from build123d import *

# Parameters (mm, degrees)
SKETCH_1_W          = 70
SKETCH_1_H          = 40
EXTRUDE_1_DEPTH     = 1.5
FILLET_1_R          = 3
SKETCH_2_W          = 13.5
SKETCH_2_H          = 20.4
CUT_EXTRUDE_1_DEPTH = 41.339186903


with BuildPart() as part:
    # Эскиз1 → Бобышка-Вытянуть1 (new body)
    with BuildSketch(Plane(origin=(0, 0, 0), x_dir=(1, 0, 0), z_dir=(0, 1, 0))):
        Rectangle(SKETCH_1_W, SKETCH_1_H)
    extrude(amount=EXTRUDE_1_DEPTH)

    # Скругление1
    fillet_1_edges = [part.edges().sort_by_distance(p)[0] for p in [
        (-35, 0.75, -20),
        (35, 0.75, -20),
        (35, 0.75, 20),
        (-35, 0.75, 20),
    ]]
    fillet(fillet_1_edges, radius=FILLET_1_R)

    # Эскиз2 → Вырез-Вытянуть1 (cut, through all)
    with BuildSketch(Plane(origin=(0, 1.5, 0), x_dir=(1, 0, 0), z_dir=(0, 1, 0))):
        with Locations((28.25, 0)):
            Rectangle(SKETCH_2_W, SKETCH_2_H)
    extrude(amount=-CUT_EXTRUDE_1_DEPTH, mode=Mode.SUBTRACT)


solid = part.part
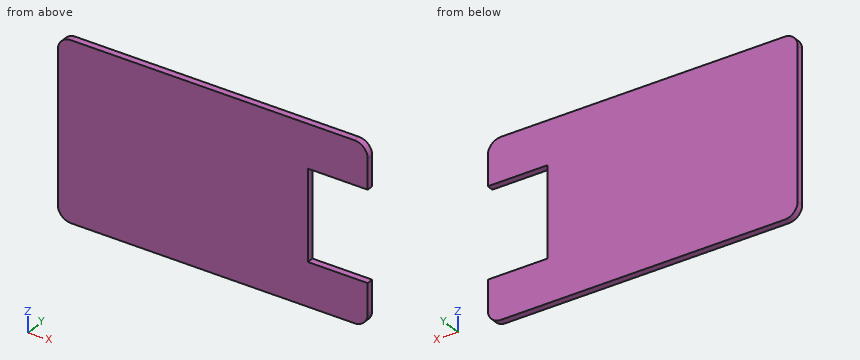
The listing builds one solid part. Answer for the finished solid, in the listing's coordinates (mm). Round coordinates to 2 decimals unless told otherwise and drop trailing zeros. Write each loop counter-clockwise with the first axis right and the second up, starting at its lowest first coordinate (ties: lowest second). Pieces come first, ordered by that corner, then holes. Notation, with made-up numbers: (-23, 74) - (-2, 74) arc R21 cw to (-2, 102) - close; hole circle Ø3 at (-9, -30). An arc over 180 degrees is marked (long way). Use a Markdown table: item, result. Add a question column.
1. Consider line 1 (Z direction, x = 27, y = 0.9); line 2 (X direction, y = 0.5, z = 0); line 3 (X direction, y = 1.2, z = 17.5). Determine where each line is inside the solid, lowest interval first.
2. The part is cut by section A-A (x = 29). Write down the section's boundary in (y, z), and give its area (3 significant figures).
3. The part is cut by section B-B (y = 1.1). Write down the section's boundary in (x, z).
4. The part is cut by section C-C (z = 8.5). Write down the section's boundary in (x, y).
Reported:
| question | item | result |
|---|---|---|
| 1 | line 1 | -20 to -10.2, 10.2 to 20 |
| 1 | line 2 | -35 to 21.5 |
| 1 | line 3 | -34.96 to 34.96 |
| 2 | outline | (0, -20) - (1.5, -20) - (1.5, -10.2) - (0, -10.2) - close; (0, 10.2) - (1.5, 10.2) - (1.5, 20) - (0, 20) - close |
| 2 | area | 29.4 mm^2 |
| 3 | outline | (-35, -17) arc R3 ccw to (-32, -20) - (32, -20) arc R3 ccw to (35, -17) - (35, -10.2) - (21.5, -10.2) - (21.5, 10.2) - (35, 10.2) - (35, 17) arc R3 ccw to (32, 20) - (-32, 20) arc R3 ccw to (-35, 17) - close |
| 4 | outline | (-35, 0) - (21.5, 0) - (21.5, 1.5) - (-35, 1.5) - close |
